Part model, mm, in its own coordinate system. Give positions to 0.01 mm unless a question says otherwise; leave off trailing zeros. Loops run counter-clockwise (first coordinate to the right, second up) from the corner with the lowest first, then second, coordinate; pieces in that order, holes last. Notation, with made-up numbers: M 71,48.25 L 130,48.25 A15 ccw 130,76.25 Z; hole C -8.5,-4.75 d1. An arc over 180 degrees is marked long. Answer in a Markdown table with one row per item.
from build123d import *

# Parameters (mm, degrees)
F1_DEPTH = 5
F2_D     = 6.3
F3_R     = 1


with BuildPart() as f1:
    # F0 (on Top) → F1 (new body)
    with BuildSketch(Plane.XY):
        Polygon((5.0011666315, 2.8847297373), (0.0023340802, 5.7735022201), (-4.9988325513, 2.8887724828), (-5.0011666315, -2.8847297373), (-0.0023340802, -5.7735022201), (4.9988325513, -2.8887724828), align=None)
    extrude(amount=F1_DEPTH)

    # F2 (through all)
    with Locations(Plane(origin=(0, 0, 0), x_dir=(1, 0, 0), z_dir=(0, 0, -1))):
        with Locations((0, 0)):
            Hole(F2_D / 2)

    # F3
    f3_edges = [f1.edges().sort_by_distance(p)[0] for p in [
        (-0.002334, -5.773502, 2.5),
        (4.998833, -2.888772, 2.5),
        (5.001167, 2.88473, 2.5),
        (0.002334, 5.773502, 2.5),
        (-4.998833, 2.888772, 2.5),
        (-5.001167, -2.88473, 2.5),
    ]]
    fillet(f3_edges, radius=F3_R)


solid = f1.part
(1) Saw through at A-A (x = 0). Write the cut outline in (y, z), plus the area to 3 significant figures.
Recorded:
| item | result |
|---|---|
| outline | M -5.62,0 L -3.15,0 L -3.15,5 L -5.62,5 Z; M 3.15,0 L 5.62,0 L 5.62,5 L 3.15,5 Z |
| area | 24.7 mm^2 |
(2) Drill centre lines: line 1 along Y through (x, z) = (0, 1.3); line 2 along X through (y, z) = (-1.25, 2.4); line 3 along X through (y, z) = (-1.5, 3.5). Where is each one in solid material? Low to high.
Recorded:
| item | result |
|---|---|
| line 1 | y = -5.62 to -3.15, 3.15 to 5.62 |
| line 2 | x = -5 to -2.89, 2.89 to 5 |
| line 3 | x = -5 to -2.77, 2.77 to 5 |
(3) Pin check, flat tips, straight feed: pin 1 Ø1 at (y, z) = (4, 4) entering from +X; pin 2 Ø1.5 at (x, z) = (-3.5, 2.5) entering from +Y. Stop position of each tip, or through.
Recorded:
| item | result |
|---|---|
| pin 1 | stops at x = 3.94 |
| pin 2 | stops at y = 4.19 |
(4) Saw through at B-B (y = 0). Write the cut outline in (x, z), plus the area to 3 significant figures.
Recorded:
| item | result |
|---|---|
| outline | M -5,0 L -3.15,0 L -3.15,5 L -5,5 Z; M 3.15,0 L 5,0 L 5,5 L 3.15,5 Z |
| area | 18.5 mm^2 |
(5) Saw through at C-C (z = 1.4). Write the cut outline in (x, y), plus the area to 3 significant figures.
Recorded:
| item | result |
|---|---|
| outline | M -5,-2.31 A1 ccw -4.5,-3.17 L -0.5,-5.48 A1 ccw 0.5,-5.49 L 4.5,-3.18 A1 ccw 5,-2.31 L 5,2.31 A1 ccw 4.5,3.17 L 0.5,5.48 A1 ccw -0.5,5.49 L -4.5,3.18 A1 ccw -5,2.31 Z; hole C 0,0 d6.3 |
| area | 55.1 mm^2 |
(6) Pull direction X, two halves, no side cores. Call faces 1 (the face through (3.3, 0.1, 0)), 2 (the face through (-2.53, -4.313, 2.465)), 3 (the face through (2.5, 1.917, 2.535)), 4 (the face through (0.01, -5.62, 2.54)): +X half, -X half, draft (parallel to the pull), parting line (faces both ways), or undercut.
Recorded:
| item | result |
|---|---|
| face 1 | draft |
| face 2 | -X half |
| face 3 | undercut |
| face 4 | parting line |
(7) Saw through at D-D (x = -4). Write the cut outline in (y, z), plus the area to 3 significant figures.
Recorded:
| item | result |
|---|---|
| outline | M -3.46,0 L 3.46,0 L 3.46,5 L -3.46,5 Z |
| area | 34.6 mm^2 |
